```python
from build123d import *

# Parameters (mm, degrees)
F0_R     = 85.979
F0_R_2   = 3.429
F0_R_3   = 6.604
F0_R_4   = 8.255
F1_DEPTH = 19.05
F2_DEPTH = 16.51
F3_DEPTH = 12.7


with BuildPart() as f1:
    # F0 (on Top) → F1 (new body)
    with BuildSketch(Plane.XY):
        Circle(F0_R)
        with Locations((-7.301313, -69.467354)):
            Circle(F0_R_2, mode=Mode.SUBTRACT)
        with Locations((-34.925, -60.491874)):
            Circle(F0_R_2, mode=Mode.SUBTRACT)
        with Locations((-56.509837, -41.0568)):
            Circle(F0_R_2, mode=Mode.SUBTRACT)
        with Locations((-68.32361, -14.522632)):
            Circle(F0_R_2, mode=Mode.SUBTRACT)
        with Locations((-38.494829, -22.225)):
            Circle(F0_R_3, mode=Mode.SUBTRACT)
        with Locations((21.584837, -66.431298)):
            Circle(F0_R_2, mode=Mode.SUBTRACT)
        with Locations((0, -44.45)):
            Circle(F0_R_3, mode=Mode.SUBTRACT)
        with Locations((46.738773, -51.908666)):
            Circle(F0_R_2, mode=Mode.SUBTRACT)
        with Locations((38.494829, -22.225)):
            Circle(F0_R_3, mode=Mode.SUBTRACT)
        with Locations((0, -19.05)):
            Circle(F0_R_4, mode=Mode.SUBTRACT)
        with Locations((63.81115, -28.410555)):
            Circle(F0_R_2, mode=Mode.SUBTRACT)
        with Locations((-68.32361, 14.522632)):
            Circle(F0_R_2, mode=Mode.SUBTRACT)
        with Locations((-56.509837, 41.0568)):
            Circle(F0_R_2, mode=Mode.SUBTRACT)
        with Locations((-16.497784, 9.525)):
            Circle(F0_R_4, mode=Mode.SUBTRACT)
        with Locations((-38.494829, 22.225)):
            Circle(F0_R_3, mode=Mode.SUBTRACT)
        with Locations((-34.925, 60.491874)):
            Circle(F0_R_2, mode=Mode.SUBTRACT)
        with Locations((-7.301313, 69.467354)):
            Circle(F0_R_2, mode=Mode.SUBTRACT)
        with Locations((16.497784, 9.525)):
            Circle(F0_R_4, mode=Mode.SUBTRACT)
        with Locations((38.494829, 22.225)):
            Circle(F0_R_3, mode=Mode.SUBTRACT)
        with Locations((69.85, 0)):
            Circle(F0_R_2, mode=Mode.SUBTRACT)
        with Locations((63.81115, 28.410555)):
            Circle(F0_R_2, mode=Mode.SUBTRACT)
        with Locations((0, 44.45)):
            Circle(F0_R_3, mode=Mode.SUBTRACT)
        with Locations((21.584837, 66.431298)):
            Circle(F0_R_2, mode=Mode.SUBTRACT)
        with Locations((46.738773, 51.908666)):
            Circle(F0_R_2, mode=Mode.SUBTRACT)
        with Locations((-68.32361, 14.522632)):
            Circle(F0_R_2)
        with Locations((-68.32361, -14.522632)):
            Circle(F0_R_2)
        with Locations((-56.509837, -41.0568)):
            Circle(F0_R_2)
        with Locations((-34.925, -60.491874)):
            Circle(F0_R_2)
        with Locations((-7.301313, -69.467354)):
            Circle(F0_R_2)
        with Locations((21.584837, -66.431298)):
            Circle(F0_R_2)
        with Locations((46.738773, -51.908666)):
            Circle(F0_R_2)
        with Locations((63.81115, -28.410555)):
            Circle(F0_R_2)
        with Locations((69.85, 0)):
            Circle(F0_R_2)
        with Locations((63.81115, 28.410555)):
            Circle(F0_R_2)
        with Locations((46.738773, 51.908666)):
            Circle(F0_R_2)
        with Locations((21.584837, 66.431298)):
            Circle(F0_R_2)
        with Locations((-7.301313, 69.467354)):
            Circle(F0_R_2)
        with Locations((-34.925, 60.491874)):
            Circle(F0_R_2)
        with Locations((-56.509837, 41.0568)):
            Circle(F0_R_2)
        with Locations((-38.494829, 22.225)):
            Circle(F0_R_3)
        with Locations((-38.494829, -22.225)):
            Circle(F0_R_3)
        with Locations((0, -44.45)):
            Circle(F0_R_3)
        with Locations((0, -19.05)):
            Circle(F0_R_4)
        with Locations((-16.497784, 9.525)):
            Circle(F0_R_4)
        with Locations((16.497784, 9.525)):
            Circle(F0_R_4)
        with Locations((38.494829, -22.225)):
            Circle(F0_R_3)
        with Locations((38.494829, 22.225)):
            Circle(F0_R_3)
        with Locations((0, 44.45)):
            Circle(F0_R_3)
    extrude(amount=-F1_DEPTH)

    # F0 (on Top) → F2 (cut)
    with BuildSketch(Plane.XY):
        with Locations((-68.32361, 14.522632)):
            Circle(F0_R_2)
        with Locations((-68.32361, -14.522632)):
            Circle(F0_R_2)
        with Locations((-56.509837, -41.0568)):
            Circle(F0_R_2)
        with Locations((-34.925, -60.491874)):
            Circle(F0_R_2)
        with Locations((-7.301313, -69.467354)):
            Circle(F0_R_2)
        with Locations((21.584837, -66.431298)):
            Circle(F0_R_2)
        with Locations((46.738773, -51.908666)):
            Circle(F0_R_2)
        with Locations((63.81115, -28.410555)):
            Circle(F0_R_2)
        with Locations((69.85, 0)):
            Circle(F0_R_2)
        with Locations((63.81115, 28.410555)):
            Circle(F0_R_2)
        with Locations((46.738773, 51.908666)):
            Circle(F0_R_2)
        with Locations((21.584837, 66.431298)):
            Circle(F0_R_2)
        with Locations((-7.301313, 69.467354)):
            Circle(F0_R_2)
        with Locations((-34.925, 60.491874)):
            Circle(F0_R_2)
        with Locations((-56.509837, 41.0568)):
            Circle(F0_R_2)
        with Locations((-38.494829, -22.225)):
            Circle(F0_R_3)
        with Locations((0, -44.45)):
            Circle(F0_R_3)
        with Locations((38.494829, -22.225)):
            Circle(F0_R_3)
        with Locations((38.494829, 22.225)):
            Circle(F0_R_3)
        with Locations((0, 44.45)):
            Circle(F0_R_3)
        with Locations((-38.494829, 22.225)):
            Circle(F0_R_3)
    extrude(amount=-F2_DEPTH, mode=Mode.SUBTRACT)

    # F0 (on Top) → F3 (cut)
    with BuildSketch(Plane.XY):
        with Locations((-16.497784, 9.525)):
            Circle(F0_R_4)
        with Locations((0, -19.05)):
            Circle(F0_R_4)
        with Locations((16.497784, 9.525)):
            Circle(F0_R_4)
    extrude(amount=-F3_DEPTH, mode=Mode.SUBTRACT)


solid = f1.part
```
Model file for the job. Use its own axes, mm. Coordinates: 2 decimals unless noted, no trailing zeros. Loops run counter-clockwise (first coordinate to the right, second up) from the corner with the lowest first, then second, coordinate; pieces in that order, holes last. Notation, with made-up numbers: M 49.5,60.5 L 55.5,60.5 A16 ccw 55.5,73.5 Z; hole C 2.25,25 d9. An arc over 180 degrees is marked long. Use CSV: the item, a comma, the result in double quotes. Start each with the question number.
1. Band-saw the part on B-B, the plane x = 0. List the corners of the cut face in (y, z) (3 decimals), then the cut area to 3 significant figures.
2. Band-saw the part on D-D, the plane x = 69.85. List the corners of the cut face in (y, z), then the cut area to 3 significant figures.
3. Band-saw the part on C-C, the plane y = 20. List the corners of the cut face in (x, z), then the cut area to 3 significant figures.
4. Band-saw the part on A-A, the plane z = -10. Give the number of separate pieces and of enclosed holes in the cut face, then the cut area to 3 significant figures.
5. Probe probe 1 along Y at (x, z) = (-0.5, -11); probe 2 along Y at (x, z) = (0, -8.75) (3 decimals); probe 3 along Y at (x, z) = (-5.5, -4.75). List the from-to ranges inside material, lowest first. Write a range as [from, to].
6. Flat gauge pins, fed straight in: pin 1 (3.5 mm diameter, centred on x = -6, y = -69, fed in from +Z); pin 2 (6 mm diameter, centred on x = -41, z = -6.5, fed in from -Y); pin 3 (1 mm diameter, centred on x = 43, z = -4.5, fed in from +Y). Where does each tip first touch, or does it go through?
7. Two-plate mould, pull along X, no slides. Class faces 1 (the flat face through (-35, 61, -16.51)), 2 (the cylindrical face through (-18.639, -83.934, -9.392)), 3 (the flat face through (-1, 1, 0)): pulls with the +X half, pulls with the -X half, needs draft (parallel to the pull), parting line crosses it, or undercut.
Entries:
1,outline,"M -85.979,-19.05 L 85.979,-19.05 L 85.979,0 L 51.054,0 L 51.054,-16.51 L 37.846,-16.51 L 37.846,0 L -10.795,0 L -10.795,-12.7 L -27.305,-12.7 L -27.305,0 L -37.846,0 L -37.846,-16.51 L -51.054,-16.51 L -51.054,0 L -85.979,0 Z"
1,area,"2,630 mm2"
2,outline,"M -50.13,-19.05 L 50.13,-19.05 L 50.13,0 L 3.43,0 L 3.43,-16.51 L -3.43,-16.51 L -3.43,0 L -50.13,0 Z"
2,area,"1,800 mm2"
3,outline,"M -83.62,-19.05 L 83.62,-19.05 L 83.62,0 L 44.71,0 L 44.71,-16.51 L 32.28,-16.51 L 32.28,0 L -32.28,0 L -32.28,-16.51 L -44.71,-16.51 L -44.71,0 L -83.62,0 Z"
3,area,"2,780 mm2"
4,separate pieces,"1"
4,enclosed holes,"24"
4,area,"21,200 mm2"
5,probe 1,"y = [-85.98, -51.04], [-37.86, -27.29], [-10.81, 37.86], [51.04, 85.98]"
5,probe 2,"y = [-85.979, -51.054], [-37.846, -27.305], [-10.795, 37.846], [51.054, 85.979]"
5,probe 3,"y = [-85.8, -72.39], [-66.55, -48.11], [-40.79, -25.21], [-12.89, 40.79], [48.11, 66.55], [72.39, 85.8]"
6,pin 1,"stops at z = -16.51"
6,pin 2,"stops at y = -77.13"
6,pin 3,"stops at y = 74.74"
7,face 1,"undercut"
7,face 2,"parting line crosses it"
7,face 3,"needs draft"
